Geometry check sheet. Reference: the model listing, model coordinates, mm. A direction names the side the tool comes from. Coordinates: 2 decimals unless noted, no trailing zeros. Order: outer loops, then holes, each group sorted by start corner. A loop starts at its lowest first (then second) coordinate and runs counter-clockwise, first axis right, second up. Notation, with made-up numbers: M 41.25,-17.75 L 78.25,-17.75 A12 ccw 78.25,-6.75 Z; hole C -6,-8.5 d10. An arc over 180 degrees is marked long. One line per item, written item: value. Start each with the question number.
1) Sectioned sample at A-A, the plane z = 7.3. Enter the section's corners in (x, y).
2) Sectioned sample at B-B, the plane x = 8. Enter the section's corners in (y, z).
3) Sectioned sample at C-C, the plane z = 5.7. Enter the section's corners in (x, y).
4) Thickness scan on L1, parallel to Z at x = 11.25, y = -1.25; L2, parallel to X at y = -1.5, z = 6.5; L3, parallel to X at y = -2, z = 6.45. Record the ranges inside material, lowest first. Write a range as from..to.
5) Go/stop test with flat-tipped pins: P1, Ø4, axis at x = 0, y = 0, coming from the -Z side; P2, Ø1.5, axis at y = -2, z = 8.5, coming from the +X side; P3, Ø1.7, axis at x = 13.5, y = 0, coming from the -Z side. Record where each tip stops, or that it passes through.
6) Access from +Z, -Z, +X, -X, +Y, -Y to the whole of each face (thin tool, end or side, straight path). Record for faces 1 (the flat face through (1, -1, 9)), 2 (the cylindrical face through (10.25, 0.03, 7.99)), 3 (the cylindrical face through (0.86, -2.08, 6.48)).
7) Sectioned sample at D-D, the plane y = 2.5. Enter the section's corners in (x, z), then the cut area to 3 significant figures.
8) Draft check along Y on faces 4 (the flat face through (8.634, 2.506, 7.986)), 5 (the cylindrical face through (7.75, 0.03, 7.99)), 6 (the flat face through (0.7, 2.3, 5)), 7 (the flat face through (8.634, -2.506, 7.986)). Enter one of: pulls with the +Y half, pulls with the -Y half, needs draft (parallel to the pull), parting line crosses it, or undercut.
```python
from build123d import *

# Parameters (mm, degrees)
PAD004_DEPTH     = 2
PAD024_DEPTH     = 1
PAD025_DEPTH     = 2
SKETCH009_R      = 2.25
POCKET023_DEPTH  = 3
REVOLUTION_ANGLE = -180


with BuildPart() as part:
    # Sketch046 → Pad004 (new body)
    with BuildSketch(Plane.XY):
        with BuildLine():
            ThreePointArc((1.2990381057, 3.25), (0.6614378278, 3.4369317712), (0, 3.5))
            Line((0, 3.5), (0, 1.25))
            ThreePointArc((1.25, 0), (0.8838834765, 0.8838834765), (0, 1.25))
            Line((1.25, 0), (5.25, 0))
            ThreePointArc((6.75, 0), (6, 0.75), (5.25, 0))
            Line((6.75, 0), (7.75, 0))
            ThreePointArc((9.25, 0), (8.5, 0.75), (7.75, 0))
            Line((9.25, 0), (10.25, 0))
            ThreePointArc((11.75, 0), (11, 0.75), (10.25, 0))
            Line((11.75, 0), (12.75, 0))
            ThreePointArc((14.25, 0), (13.5, 0.75), (12.75, 0))
            Line((14.25, 0), (15.25, 0))
            ThreePointArc((16.75, 0), (16, 0.75), (15.25, 0))
            Line((16.75, 0), (17.75, 0))
            ThreePointArc((17.75, 0), (17.2983689647, 1.1733448051), (16.1765851067, 1.7410679769))
            Line((1.2990381057, 3.25), (16.1765851067, 1.7410679769))
        make_face()
    extrude(amount=PAD004_DEPTH)

    # Sketch047 → Pad024 (join)
    with BuildSketch(Plane.XY.offset(2)):
        with BuildLine():
            ThreePointArc((3.5, 0), (2.4748737342, 2.4748737342), (0, 3.5))
            Line((0, 3.5), (0, 2.25))
            ThreePointArc((2.25, 0), (1.5909902577, 1.5909902577), (0, 2.25))
            Line((2.25, 0), (3.5, 0))
        make_face()
    extrude(amount=PAD024_DEPTH)

    # Sketch048 → Pad025 (join)
    with BuildSketch(Plane.XY):
        with BuildLine():
            ThreePointArc((3.5, 0), (2.4748737342, 2.4748737342), (0, 3.5))
            Line((0, 3.5), (0, 1.25))
            ThreePointArc((1.25, 0), (0.8838834765, 0.8838834765), (0, 1.25))
            Line((3.5, 0), (1.25, 0))
        make_face()
    extrude(amount=-PAD025_DEPTH)

    # Sketch009 → Pocket023 (cut)
    with BuildSketch(Plane.XY.offset(-2)):
        Circle(SKETCH009_R)
    extrude(amount=POCKET023_DEPTH, mode=Mode.SUBTRACT)

    # Mirrored009: part across Sketch009 H_Axis


with BuildPart() as part_1:
    add(part.part)
    add(part.part.mirror(Plane(origin=(0, 0, -2), x_dir=(0, 0, 1), z_dir=(0, 1, 0))))

    # Mirrored009 Face3 → Revolution (revolve)
    with BuildSketch(Plane(origin=(0, -2.7198275862, 0.6379310345), x_dir=(0, 1, 0), z_dir=(-1, 0, 0))):
        Polygon((0.4698275862, 2.6379310345), (-0.7801724138, 2.6379310345), (-0.7801724138, -2.3620689655), (0.4698275862, -2.3620689655), (0.4698275862, -1.3620689655), (1.4698275862, -1.3620689655), (1.4698275862, -0.3620689655), (0.4698275862, -0.3620689655), align=None)
    revolve(axis=Axis((0, 0, 0), (0, 0, 1)), revolution_arc=REVOLUTION_ANGLE)


with BuildPart() as part_2:
    # Body002 placement: moved
    add(part_1.part.moved(Location((0, 0, 7))))


solid = part_2.part
```
Final values:
1. outline: M 1.3,-3.25 L 16.18,-1.74 A1.75 ccw 16.18,1.74 L 1.3,3.25 A3.5 ccw long Z; hole C 0,0 d4.5; hole C 6,0 d1.5; hole C 8.5,0 d1.5; hole C 11,0 d1.5; hole C 13.5,0 d1.5; hole C 16,0 d1.5
2. outline: M -2.57,7 L -0.56,7 L -0.56,9 L -2.57,9 Z; M 0.56,7 L 2.57,7 L 2.57,9 L 0.56,9 Z
3. outline: C 0,0 d7; hole C 0,0 d4.5
4. L1: z = 7..9
4. L2: x = -3.16..-1.68, 1.68..3.16
4. L3: x = -2.87..-1.03, 1.03..2.87
5. P1: stops at z = 8
5. P2: stops at x = 17.22
5. P3: stops at z = 7
6. face 1: +Z
6. face 2: +Z, -Z
6. face 3: -Z
7. outline: M -2.45,5 L 2.45,5 L 2.45,7 L 8.69,7 L 8.69,9 L 2.45,9 L 2.45,10 L -2.45,10 Z
7. area: 37.0 mm^2
8. face 4: pulls with the +Y half
8. face 5: undercut
8. face 6: needs draft
8. face 7: pulls with the -Y half
